CAD build for the part. Positions are in the model's coordinates, mm. Face numbers are marked on the shaded views. Coordinates: 2 decimals unless noted, no trailing zeros. Order: outer loops, then holes, each group sorted by start corner. A loop starts at its lowest first (then second) coordinate and runs counter-clockwise, first axis right, second up. Notation, with made-up numbers: M -17.75,12 L 11.25,12 A16 cw 11.25,43 Z; hole C 48,17 d9. An arc over 180 degrees is marked long. Write item = value, one per line.
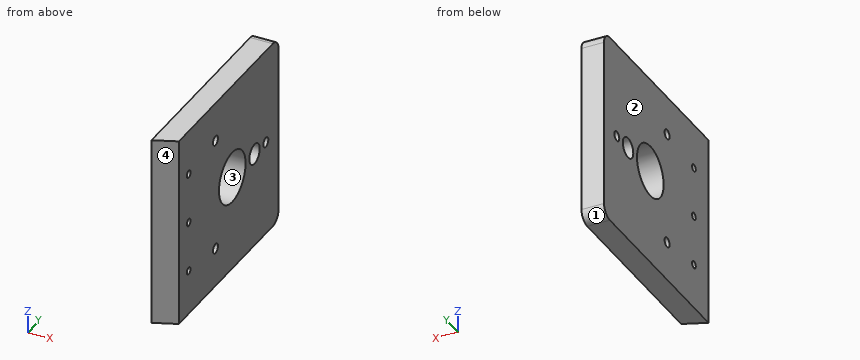
from build123d import *

# Parameters (mm, degrees)
BOSS_EXTRUDE1_DEPTH = 85
SKETCH3_R           = 11.5
SKETCH3_R_2         = 4.5
SKETCH3_R_3         = 2.15
CUT_EXTRUDE1_DEPTH  = 85
SKETCH4_R           = 1.6
CUT_EXTRUDE2_DEPTH  = 85
FILLET1_R           = 5


with BuildPart() as part:
    # Sketch2 → Boss-Extrude1 (new body)
    with BuildSketch(Plane.XY):
        Polygon((0, 0), (0, 86.2), (-10, 86.2), (-10, -4.142135624), align=None)
    extrude(amount=BOSS_EXTRUDE1_DEPTH)

    # Sketch3 → Cut-Extrude1 (cut)
    with BuildSketch(Plane.ZY.offset(10)):
        with Locations(Location((42.5, 46.2, 0), (0, 0, 270))):
            Circle(SKETCH3_R)
        with Locations(Location((42.5, 65.45, 0), (0, 0, 270))):
            Circle(SKETCH3_R_2)
        with Locations(Location((42.5, 75.2, 0), (0, 0, 270))):
            Circle(SKETCH3_R_3)
        with Locations(Location((67.61473671, 31.7, 0), (0, 0, 270))):
            Circle(SKETCH3_R_3)
        with Locations(Location((17.38526329, 31.7, 0), (0, 0, 270))):
            Circle(SKETCH3_R_3)
    extrude(amount=-CUT_EXTRUDE1_DEPTH, mode=Mode.SUBTRACT)

    # Sketch4 → Cut-Extrude2 (cut)
    with BuildSketch(Plane(origin=(0, 0, 0), x_dir=(0, 0, -1), z_dir=(1, 0, 0))):
        with Locations((-65, 8.5)):
            Circle(SKETCH4_R)
        with Locations((-20, 8.5)):
            Circle(SKETCH4_R)
        with Locations((-42.5, 8.5)):
            Circle(SKETCH4_R)
    extrude(amount=-CUT_EXTRUDE2_DEPTH, mode=Mode.SUBTRACT)

    # Fillet1
    fillet1_edges = [part.edges().sort_by_distance(p)[0] for p in [
        (-5, 86.2, 85),
        (-5, 86.2, 0),
    ]]
    fillet(fillet1_edges, radius=FILLET1_R)


solid = part.part
(1) Wall check: line 1 (Z direction, x = -3, y = 31.7); line 2 (Z direction, x = -7.5, y = 65.45); line 3 (Y direction, x = -6.5, z = 41.5). Give the ranges that are in metal, low to high. Write a range as from..to.
Evaluation:
line_1 = 0..15.24, 19.54..65.46, 69.76..85
line_2 = 0..38, 47..85
line_3 = -2.69..7.25, 9.75..34.74, 57.66..61.06, 69.84..73.3, 77.1..86.2
(2) Slice it at B-B, the plane z = 51. Write the cut outline in (x, y).
Evaluation:
outline = M -10,-4.14 L 0,0 L 0,38.45 L -10,38.45 Z; M -10,53.95 L 0,53.95 L 0,86.2 L -10,86.2 Z
(3) Pull direction Y, two halves, no side cores. Call the marked faces 1, 2, 3 and 4: +Y half, -Y half, draft (parallel to the pull), parting line (faces both ways), or undercut.
Evaluation:
face_1 = +Y half
face_2 = draft
face_3 = undercut
face_4 = -Y half
(4) Slice it at D-D, the plane x = -8.5. State how many separate pieces and enclosed holes the cut face has, then the cut area to 3 significant figures.
Evaluation:
separate_pieces = 1
enclosed_holes = 8
area = 7,070 mm²
(5) Slice it at C-C, the plane y = 31.7. Write the cut outline in (x, z), then the cut area to 3 significant figures.
Evaluation:
outline = M -10,0 L 0,0 L 0,15.24 L -10,15.24 Z; M -10,19.54 L 0,19.54 L 0,65.46 L -10,65.46 Z; M -10,69.76 L 0,69.76 L 0,85 L -10,85 Z
area = 764 mm²
(6) Pin check, flat tip, straight feed: pin 1 Ø4 at (y, z) = (31.7, 67.61) entering from -X. Stop position of the tip, or through.
Evaluation:
pin_1 = through
(7) Slice it at A-A, the plane y = 65.45. Write the cut outline in (x, z).
Evaluation:
outline = M -10,0 L 0,0 L 0,38 L -10,38 Z; M -10,47 L 0,47 L 0,85 L -10,85 Z
